Part model, mm, in its own coordinate system. Give positions to 0.01 mm unless a question says otherwise; leave off trailing zeros. Order: outer loops, then holes, each group sorted by start corner. A loop starts at its lowest first (then second) coordinate and runs counter-clockwise, first axis right, second up.
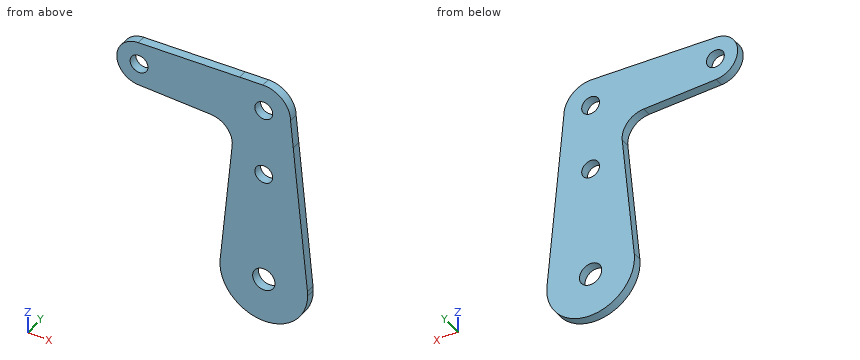
from build123d import *

# Parameters (mm, degrees)
F0_R     = 3.175
F0_R_2   = 3.96875
F1_DEPTH = 3.175
F2_R     = 7.9375


with BuildPart() as f1:
    # F0 (on Front) → F1 (new body)
    with BuildSketch(Plane.XZ):
        with BuildLine():
            ThreePointArc((-0.3401787076, -9.5189234395), (6.6138272887, -6.8544083329), (9.525, 0))
            ThreePointArc((9.525, 0), (6.6138273092, 6.8544083132), (-0.3401786508, 9.5189234415))
            ThreePointArc((-0.3401786508, 9.5189234415), (-6.5286581765, 6.9355783763), (-9.481007181, 0.9144002588))
            ThreePointArc((-9.481007181, 0.9144002588), (-7.164320199, -6.2767938541), (-0.3401787076, -9.5189234395))
        make_face()
        Circle(F0_R, mode=Mode.SUBTRACT)
        with BuildLine():
            Line((10.4874381875, -9.9058708993), (9.525, 0))
            ThreePointArc((9.525, 0), (6.6138272887, -6.8544083329), (-0.3401787076, -9.5189234395))
            Line((-0.3401787076, -9.5189234395), (10.4874381875, -9.9058708993))
        make_face()
        with BuildLine():
            ThreePointArc((-9.481007181, 0.9144002588), (-6.5286581765, 6.9355783763), (-0.3401786508, 9.5189234415))
            Line((-0.3401786508, 9.5189234415), (-8.6798843665, 9.2208866737))
            Line((-8.6798843665, 9.2208866737), (-9.481007181, 0.9144002588))
        make_face()
        with BuildLine():
            Line((-10.4524001899, -9.157542126), (-0.3401787076, -9.5189234395))
            ThreePointArc((-0.3401787076, -9.5189234395), (-7.164320199, -6.2767938541), (-9.481007181, 0.9144002588))
            Line((-9.481007181, 0.9144002588), (-10.4524001899, -9.157542126))
        make_face()
        with BuildLine():
            Line((10.4874381875, -9.9058708993), (-0.3401787076, -9.5189234395))
            Line((-0.3401787076, -9.5189234395), (-10.4524001899, -9.157542126))
            Line((-10.4524001899, -9.157542126), (-15.5488517247, -62.0003830342))
            ThreePointArc((-15.5488517247, -62.0003830342), (-0.0055160109, -47.8790009739), (15.5477887724, -61.9894023403))
            Line((15.5477887724, -61.9894023403), (10.4874381875, -9.9058708993))
        make_face()
        with Locations((0, -23.9574573934)):
            Circle(F0_R, mode=Mode.SUBTRACT)
        with BuildLine():
            Line((-10.4524001899, -9.157542126), (-9.481007181, 0.9144002588))
            Line((-9.481007181, 0.9144002588), (-8.6798843665, 9.2208866737))
            Line((-8.6798843665, 9.2208866737), (-44.7334816061, 7.9324362228))
            ThreePointArc((-44.7334816061, 7.9324362228), (-38.9384770253, 5.7120067182), (-36.5125, 0))
            ThreePointArc((-36.5125, 0), (-38.9384772211, -5.7120069072), (-44.7334821499, -7.9324362034))
            Line((-44.7334821499, -7.9324362034), (-10.4524001899, -9.157542126))
        make_face()
        with BuildLine():
            ThreePointArc((15.621, -63.5), (15.602686458, -62.7438146435), (15.5477887724, -61.9894023403))
            ThreePointArc((15.5477887724, -61.9894023403), (-0.0055160109, -47.8790009739), (-15.5488517247, -62.0003830342))
            ThreePointArc((-15.5488517247, -62.0003830342), (-0.7506757652, -79.1029525057), (15.621, -63.5))
        make_face()
        with Locations((0, -63.5)):
            Circle(F0_R_2, mode=Mode.SUBTRACT)
        with BuildLine():
            ThreePointArc((-36.5125, 0), (-38.9384770253, 5.7120067182), (-44.7334816061, 7.9324362228))
            ThreePointArc((-44.7334816061, 7.9324362228), (-52.3875, 2.721e-07), (-44.7334821499, -7.9324362034))
            ThreePointArc((-44.7334821499, -7.9324362034), (-38.9384772211, -5.7120069072), (-36.5125, 0))
        make_face()
        with Locations((-44.45, 0)):
            Circle(F0_R, mode=Mode.SUBTRACT)
    extrude(amount=F1_DEPTH)

    # F2
    f2_edges = [f1.edges().sort_by_distance(p)[0] for p in [
        (-10.4524, -1.5875, -9.157542),
    ]]
    fillet(f2_edges, radius=F2_R)


solid = f1.part
Item 1: Band-saw the part on C-C on x = 8. List the corners of the cut face in (y, z) (3 decimals).
Item 2: Band-saw the part on A-A on y = -1.55. Give the number of separate pieces and of enclosed holes in the cut face, plus the area to 3 significant figures.
Item 3: Drill centre lines: probe 1 along Z at (x, y) = (0, -2.3) (3 decimals); probe 2 along Z at (x, y) = (-44.45, -1.75) (3 decimals); probe 3 along X at (y, z) = (-1.45, 0.5). Where is each one in solid material? Low to high.
Item 4: Band-saw the part on B-B on x = -33. List the corners of the cut face in (y, z) (3 decimals), plus the area to 3 significant figures.
Item 5: Drop flat-ended pins along their axis: P1, Ø7, axis at x = 0, z = -63.5, coming from the +Y side; P2, Ø1, axis at y = -2.5, z = -68.5, coming from the -X side; P3, Ø1.5, axis at x = 6.5, y = -1, coming from the +Z side. Give the stop position or say it passes through.
Working result:
1. outline: (-3.175, -76.917) - (0, -76.917) - (0, 5.17) - (-3.175, 5.17) - close
2. separate pieces: 1
2. enclosed holes: 4
2. area: 2,710 mm2
3. probe 1: z = -79.121 to -67.469, -59.531 to -27.132, -20.782 to -3.175, 3.175 to 9.525
3. probe 2: z = -7.943 to -3.175, 3.175 to 7.943
3. probe 3: x = -52.37 to -47.59, -41.31 to -3.14, 3.14 to 9.51
4. outline: (-3.175, -8.352) - (0, -8.352) - (0, 8.352) - (-3.175, 8.352) - close
4. area: 53.0 mm2
5. P1: passes through
5. P2: stops at x = -14.96
5. P3: stops at z = 7.59
